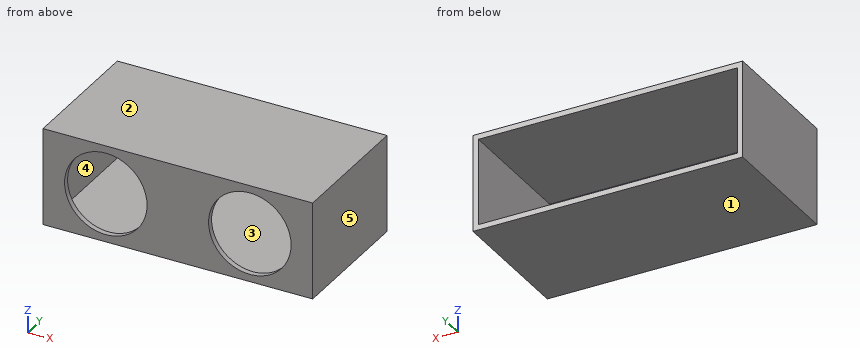
from build123d import *

# Parameters (mm, degrees)
F0_W     = 500
F0_H     = 180
F1_DEPTH = 250
F2_T     = -10
F3_R     = 76.5
F4_DEPTH = 25


with BuildPart() as f1:
    # F0 (on Front) → F1 (new body)
    with BuildSketch(Plane.XZ):
        with Locations((16.63438, -3.742575)):
            Rectangle(F0_W, F0_H)
    extrude(amount=F1_DEPTH)

    # F2
    f2_openings = [f1.faces().sort_by_distance(p)[0] for p in [
        (16.63438, 0, -3.742575),
    ]]
    offset(amount=F2_T, openings=f2_openings)

    # F3 (on face) → F4 (cut)
    with BuildSketch(Plane.XZ.offset(250)):
        with Locations((-116.86562, -3.742575)):
            Circle(F3_R)
        with Locations((150.13438, -3.742575)):
            Circle(F3_R)
    extrude(amount=-F4_DEPTH, mode=Mode.SUBTRACT)


solid = f1.part
Input: part model. Units: mm. Frame: model coordinates. Face numbers are marked on the shaded views. A direction names the side the tool comes from. Coordinates: 2 decimals unless noted, no trailing zeros. Loops run counter-clockwise (first coordinate to the right, second up) from the corner with the lowest first, then second, coordinate; pieces in that order, holes last. Notation, with made-up numbers: (37.5, -21) - (95.5, -21) arc R23 ccw to (95.5, -2) - close; hole circle Ø7 at (-19, 72). An arc over 180 degrees is marked (long way). Answer in a Markdown table with one row per item. Add a question column.
Item 1: Section query C-C on x = 61.5. Return the cut outline in (y, z), then the cut area to 3 significant figures.
Item 2: Section query B-B on z = -27. Return the cut outline in (x, y), then the cut area to 3 significant figures.
Item 3: Section query D-D on x = -160.5. Return the cut outline in (y, z), then the cut area to 3 significant figures.
Item 4: Line query: line 1 along Z through (x, y) = (-81, -42); line 2 along X through (y, z) = (-81.5, -15.5); line 3 along Y through (x, z) = (38, 40). Output: solid intervals per line, ascending. Write a range as [from, to].
Item 5: Contact query for a flat-ended pin moving along its axis: P1, Ø4, axis at x = -43.5, z = 13.5, coming from the +Y side. Output: stop coordinate, or through.
Item 6: Access query for the marked faces 4 and 5. Directions: +Z, -Z, +X, -X, +Y, -Y. A direction counts if a zero-diameter tool reaches every point of the face in a straight line with its end or side. Return the directions, or none.
Item 7: Mould query, pull axis Z, two halves, no side actions, for the marked faces 1, 2 and 3. Classes: released by +Z, released by -Z, zero draft, split by the parting line, or undercut.
Item 8: Section query A-A on y = -75.5. Return the cut outline in (x, z).
Recorded:
| question | item | result |
|---|---|---|
| 1 | outline | (-250, -93.74) - (0, -93.74) - (0, -83.74) - (-240, -83.74) - (-240, 76.26) - (0, 76.26) - (0, 86.26) - (-250, 86.26) - close |
| 1 | area | 6,600 mm^2 |
| 2 | outline | (-233.37, -250) - (-189.74, -250) - (-189.74, -240) - (-223.37, -240) - (-223.37, 0) - (-233.37, 0) - close; (-43.99, -250) - (77.26, -250) - (77.26, -240) - (-43.99, -240) - close; (223.01, -250) - (266.63, -250) - (266.63, 0) - (256.63, 0) - (256.63, -240) - (223.01, -240) - close |
| 2 | area | 6,880 mm^2 |
| 3 | outline | (-250, -93.74) - (0, -93.74) - (0, -83.74) - (-240, -83.74) - (-240, -66.58) - (-250, -66.58) - close; (-250, 59.09) - (-240, 59.09) - (-240, 76.26) - (0, 76.26) - (0, 86.26) - (-250, 86.26) - close |
| 3 | area | 5,340 mm^2 |
| 4 | line 1 | [-93.74, -83.74], [76.26, 86.26] |
| 4 | line 2 | [-233.37, -223.37], [256.63, 266.63] |
| 4 | line 3 | [-250, -240] |
| 5 | P1 | y = -240 |
| 6 | face 4 | +Y |
| 6 | face 5 | +Z, -Z, +X, +Y, -Y |
| 7 | face 1 | released by -Z |
| 7 | face 2 | released by +Z |
| 7 | face 3 | undercut |
| 8 | outline | (-233.37, -93.74) - (266.63, -93.74) - (266.63, 86.26) - (-233.37, 86.26) - close; hole (-223.37, -83.74) - (256.63, -83.74) - (256.63, 76.26) - (-223.37, 76.26) - close |
